Autodesk Inventor part; units mm, degrees
ref_plane "YZ Plane" through (0, 0, 0) normal (1, 0, 0) x (0, 1, 0)
ref_plane "XZ Plane" through (0, 0, 0) normal (0, 1, 0) x (-1, 0, 0)
ref_plane "XY Plane" through (0, 0, 0) normal (0, 0, 1) x (1, 0, 0)
sketch "Náčrt1" plane through (0, 0, 0) normal (1, 0, 0) x (0, 1, 0)
  line L0 (0, 0) -> (2.6, 0)
  line L1 (2.6, 0) -> (2.6, -28.6)
  line L2 (2.6, -28.6) -> (0, -28.6)
  line L3 (0, -28.6) -> (0, 0)
  dimension "d0" = 2.6
  dimension "d1" = 28.6
extrude "Vysunutí1" add sketch "Náčrt1" along normal blind 2.5
sketch "Náčrt2" plane through (2.5, 0, 0) normal (1, 0, 0) x (0, 0, -1)
  line L0 (-1.2, -1.2) -> (29.8, -1.2)
  line L1 (29.8, -1.2) -> (29.8, 3.8)
  line L2 (29.8, 3.8) -> (-1.2, 3.8)
  line L3 (-1.2, 3.8) -> (-1.2, -1.2)
  line L4 (-1.2, -1.2) -> (29.8, 3.8) construction
  line L5 (29.8, -1.2) -> (-1.2, 3.8) construction
  line L6 (28.6, 2.6) -> (0, 2.6)
  point P0 (0, 0)
  point P1 (14.3, 1.3)
  dimension "d4" = 31
  dimension "d5" = 5
  dimension "d6" = 1.2
extrude "Vysunutí2" add sketch "Náčrt2" along normal blind 1
properties part number "CardCover"
Design review of the part built by this model. Coordinates are the model's own, in mm. A direction names the side the tool comes from. Give positions to 0.01 mm unless a question says otherwise; leave off trailing zeros. Order: outer loops, then holes, each group sorted by start corner. A loop starts at its lowest first (then second) coordinate and runs counter-clockwise, first axis right, second up. Notation, with made-up numbers: M 29,78 L 85,78 A21 ccw 85,85 Z; hole C -7.5,14.5 d7. An arc over 180 degrees is marked long. One line per question, with ' | ' between items. Start each with the question number.
Q1. We need section A-A (z = -2). Write out the cut boundary in (x, y).
Q2. We need section B-B (y = 1.25). Write out the cut boundary in (x, z).
Q3. For pin 1 Ø2 at (x, y) = (1, 1) entering from -Z; pin 2 Ø0.8 at (x, z) = (2, -18.5) entering from +Y, all flat-tipped, find the tip position at first contact; note any pin that passes through.
Q4. For L1, parallel to Z at x = 0.65, y = 2.05; L2, parallel to X at y = -0.1, z = -28; L3, parallel to Y at x = 1.55, z = -26, list the stretches that pass through material, from the lowest coordinate up. Write a range as [from, to].
Q5. We need section C-C (x = 0.9). Write out the cut boundary in (y, z), plus the area to 3 significant figures.
Q6. Machinability: for faces 1 (the face through (1, 1, 0)), 2 (the face through (1, 1, -28.6)), 3 (the face through (1, 0, -15)), which of the approach directions +Z, -Z, +X, -X, +Y, -Y give a long, thin tool a straight path to every point of the face, cutting with its end or side? Answer none if there is none.
Q7. We need section D-D (y = 2.9). Write out the cut boundary in (x, z).
Returned:
1) outline: M 0,0 L 2.5,0 L 2.5,-1.2 L 3.5,-1.2 L 3.5,3.8 L 2.5,3.8 L 2.5,2.6 L 0,2.6 Z
2) outline: M 0,-28.6 L 2.5,-28.6 L 2.5,-29.8 L 3.5,-29.8 L 3.5,1.2 L 2.5,1.2 L 2.5,0 L 0,0 Z
3) pin 1: z = -28.6 | pin 2: y = 2.6
4) L1: [-28.6, 0] | L2: [2.5, 3.5] | L3: [0, 2.6]
5) outline: M 0,-28.6 L 2.6,-28.6 L 2.6,0 L 0,0 Z | area: 74.4 mm2
6) face 1: +Z, -X, +Y, -Y | face 2: -Z, -X, +Y, -Y | face 3: +Z, -Z, -X, -Y
7) outline: M 2.5,-29.8 L 3.5,-29.8 L 3.5,1.2 L 2.5,1.2 Z
